```python
from build123d import *

# Parameters (mm, degrees)
ESQUISSE1_W                      = 18
ESQUISSE1_H                      = 42
ESQUISSE2_R                      = 24
EXTRUSION1_DEPTH                 = 21
EXTRUSION2_START                 = 87
ESQUISSE3_R                      = 24
EXTRUSION2_DEPTH                 = 87
DIAM_TRE_DU_PER_AGE_M10_0_10_1_D = 10
DIAM_TRE_DU_PER_AGE_M10_0_10_2_D = 10
DIAM_TRE_DU_PER_AGE_M10_0_10_3_D = 10
PER_AGE1_D                       = 24
PER_AGE1_CBORE_D                 = 36
PER_AGE1_CBORE_DEPTH             = 99
CHANFREIN1_SIZE                  = 1


with BuildPart() as part:
    # Esquisse1 → Révolution1 (revolve)
    with BuildSketch(Plane.XY, mode=Mode.PRIVATE) as r_volution1_sk:
        with Locations((30, 21)):
            Rectangle(ESQUISSE1_W, ESQUISSE1_H)
    revolve(r_volution1_sk.sketch.rotate(Axis((21, 0, 0), (1, 0, 0)), 270), axis=Axis((21, 0, 0), (1, 0, 0)))

    # Esquisse2 → Extrusion1 (add)
    with BuildSketch(Plane.ZY.offset(-21)):
        with Locations(Location((0, 0, 0), (0, 0, 180))):
            Circle(ESQUISSE2_R)
    extrude(amount=EXTRUSION1_DEPTH)

    # Esquisse3 → Extrusion2 (add)
    with BuildSketch(Plane(origin=(39, 0, 0), x_dir=(0, 0, -1), z_dir=(1, 0, 0)).offset(EXTRUSION2_START)):
        Circle(ESQUISSE3_R)
    extrude(amount=-EXTRUSION2_DEPTH)

    # Diamètre du perçage M10.0 (10)1 (through all)
    with Locations(Plane(origin=(39, 0, 0), x_dir=(0, 0, -1), z_dir=(1, 0, 0))):
        with Locations((25.633132295, -15.586613768)):
            Hole(DIAM_TRE_DU_PER_AGE_M10_0_10_1_D / 2)

    # Diamètre du perçage M10.0 (10)2 (through all)
    with Locations(Plane(origin=(39, 0, 0), x_dir=(0, 0, -1), z_dir=(1, 0, 0))):
        with Locations((0.681837335, 29.99225063)):
            Hole(DIAM_TRE_DU_PER_AGE_M10_0_10_2_D / 2)

    # Diamètre du perçage M10.0 (10)3 (through all)
    with Locations(Plane(origin=(39, 0, 0), x_dir=(0, 0, -1), z_dir=(1, 0, 0))):
        with Locations((-26.31496963, -14.405636862)):
            Hole(DIAM_TRE_DU_PER_AGE_M10_0_10_3_D / 2)

    # Perçage1 (through all)
    with Locations(Plane.ZY):
        with Locations((0, 0)):
            CounterBoreHole(PER_AGE1_D / 2, PER_AGE1_CBORE_D / 2, PER_AGE1_CBORE_DEPTH)

    # Chanfrein1
    chanfrein1_edges = [part.edges().sort_by_distance(p)[0] for p in [
        (126, 0, 24),
        (0, 0, 24),
    ]]
    chamfer(chanfrein1_edges, length=CHANFREIN1_SIZE)


solid = part.part
```
Geometry check sheet. Reference: the model listing, model coordinates, mm. A direction names the side the tool comes from. Give positions to 0.01 mm unless a question says otherwise; leave off trailing zeros. Order: outer loops, then holes, each group sorted by start corner. A loop starts at its lowest first (then second) coordinate and runs counter-clockwise, first axis right, second up. Notation, with made-up numbers: (58.5, 68) - (68.5, 68) arc R24 ccw to (68.5, 103) - close; hole circle Ø9 at (1.5, 6.25). An arc over 180 degrees is marked (long way). Answer in a Markdown table with one row per item. Add a question column.
Q1. Cross-section at B-B, the plane z = 0. Enter the section's corners in (x, y), then the cut area to 3 significant figures.
Q2. Material ranges on probe 1 along X at (y, z) = (-24, 31.5); probe 2 along X at (y, z) = (2.5, 12.5); probe 3 along Z at (x, y) = (22, -12), recorded low to high. Write a range as from..to.
Q3. Cross-section at C-C, the plane x = 51.5. Enter the section's corners in (y, z), then the cut area to 3 significant figures.
Q4. Cross-section at A-A, the plane y = 0. Enter the section's corners in (x, z).
Q5. Cross-section at D-D, the plane y = 32.5. Enter the section's corners in (x, z), then the cut area to 3 significant figures.
Q6. Tool access check on faces 1 (the cylindrical face through (30.13, 12.62, -40.06)), 2 (the flat face through (39, -18, 18)), 3 (the cylindrical face through (11.14, -7.21, -22.89)). Record the directions out of +Z, -Z, +X, -X, +Y, -Y that give a thin tool (end or side, any length) a straight path to the whole face; none if there is none.
Q7. Mould release check, pull along Z, two halves, no side actions. Record for faces 4 (the flat face through (0, 12, 14)), 5 (the cylindrical face through (82.602, 1.055, 23.977)), 6 (the cylindrical face through (48.807, 17.847, -2.343)): pulls with the +Z half, pulls with the -Z half, needs draft (parallel to the pull), parting line crosses it, or undercut.
Q8. Gauge pin test, flat ends, axial feed: pin 1 (10 mm diameter, centred on x = 41.5, z = -22, fed in from +Y); pin 2 (5 mm diameter, centred on x = 27, z = 0.5, fed in from +Y); pin 3 (8 mm diameter, centred on x = 24.5, z = -13.5, fed in from -Y). Record the tip position at first contact, or that the pin passes through.
Check values:
| question | item | result |
|---|---|---|
| 1 | outline | (0, -23) - (1, -24) - (21, -24) - (21, -42) - (39, -42) - (39, -24) - (125, -24) - (126, -23) - (126, -12) - (99, -12) - (99, -18) - (0, -18) - close; (0, 18) - (99, 18) - (99, 12) - (126, 12) - (126, 23) - (125, 24) - (39, 24) - (39, 25.04) - (21, 25.04) - (21, 24) - (1, 24) - (0, 23) - close; (21, 34.95) - (39, 34.95) - (39, 42) - (21, 42) - close |
| 1 | area | 2,300 mm^2 |
| 2 | probe 1 | x = 21..39 |
| 2 | probe 2 | x = 99..126 |
| 2 | probe 3 | z = -40.25..-29.12, -22.15..-13.42, 13.42..21.93, 30.7..40.25 |
| 3 | outline | circle Ø48 at (0, 0); hole circle Ø36 at (0, 0) |
| 3 | area | 792 mm^2 |
| 4 | outline | (0, -23) - (1, -24) - (21, -24) - (21, -42) - (39, -42) - (39, -24) - (125, -24) - (126, -23) - (126, -12) - (99, -12) - (99, -18) - (0, -18) - close; (0, 18) - (99, 18) - (99, 12) - (126, 12) - (126, 23) - (125, 24) - (39, 24) - (39, 42) - (21, 42) - (21, 24) - (1, 24) - (0, 23) - close |
| 5 | outline | (21, -26.6) - (39, -26.6) - (39, -5.01) - (21, -5.01) - close; (21, 3.64) - (39, 3.64) - (39, 26.6) - (21, 26.6) - close |
| 5 | area | 802 mm^2 |
| 6 | face 1 | +X, -X |
| 6 | face 2 | +X |
| 6 | face 3 | -X |
| 7 | face 4 | needs draft |
| 7 | face 5 | parting line crosses it |
| 7 | face 6 | undercut |
| 8 | pin 1 | stops at y = 38.1 |
| 8 | pin 2 | stops at y = 42 |
| 8 | pin 3 | stops at y = -40.91 |
